from build123d import *

# Parameters (mm, degrees)
F0_R     = 5
F1_DEPTH = 10


with BuildPart() as f1:
    # F0 (on Top) → F1 (new body, symmetric)
    with BuildSketch(Plane.XY):
        with BuildLine():
            Line((25, 25), (25, 10))
            Line((25, 10), (-25, 10))
            ThreePointArc((-25, 10), (-35, 0), (-25, -10))
            Line((-25, -10), (25, -10))
            Line((25, -10), (25, -25))
            ThreePointArc((25, -25), (35, -35), (45, -25))
            Line((45, -25), (45, 25))
            ThreePointArc((45, 25), (35, 35), (25, 25))
        make_face()
        with Locations((35, -25)):
            Circle(F0_R, mode=Mode.SUBTRACT)
        with Locations((-25, 0)):
            Circle(F0_R, mode=Mode.SUBTRACT)
        with Locations((25, 0)):
            Circle(F0_R, mode=Mode.SUBTRACT)
        with Locations((35, 25)):
            Circle(F0_R, mode=Mode.SUBTRACT)
    extrude(amount=F1_DEPTH, both=True)


solid = f1.part
CAD build for the part. Positions are in the model's coordinates, mm. A direction names the side the tool comes from. Give positions to 0.01 mm unless a question says otherwise; leave off trailing zeros. Loops run counter-clockwise (first coordinate to the right, second up) from the corner with the lowest first, then second, coordinate; pieces in that order, holes last. Notation, with made-up numbers: M -29,49.5 L -10,49.5 A36 cw -10,86.5 Z; hole C -15,2.25 d3. An arc over 180 degrees is marked long. One line per question, with ' | ' between items. Start each with the question number.
1. Saw through at B-B on y = -21. Give the cut face in (x, z), plus the area to 3 significant figures.
2. Saw through at C-C on x = 21.5. Give the cut face in (y, z), plus the area to 3 significant figures.
3. Probe L1, parallel to Y at x = -25, z = 3.25; L2, parallel to X at y = -1, z = 2.75; L3, parallel to Y at x = 29.5, z = 7.25. List the from-to ranges inside material, lowest first. Write a range as from..to.
4. Flat gauge pins, fed straight in: pin 1 (4.5 mm diameter, centred on y = -19, z = -0.5, fed in from -X); pin 2 (8 mm diameter, centred on x = 1, z = -7.5, fed in from +Y); pin 3 (10 mm diameter, centred on x = 1.5, z = 0.5, fed in from -Y). Where does each tip first touch, or does it go through?
5. Two-plate mould, pull along Y, no slides. Class faces 4 (the face through (-35, 0, 0)), 5 (the face through (31, 22, 0)), 6 (the face through (25, 18, 0)), 7 (the face through (31, -28, 0)): pulls with the +Y half, pulls with the -Y half, needs draft (parallel to the pull), parting line crosses it, or undercut.
6. Saw through at A-A on y = 0. Give the cut face in (x, z), plus the area to 3 significant figures.
7. 3-axis set-ups, long thin cutter, end or side, ignore diameter. For faces 1 (the face through (0, -10, 0)), 2 (the face through (45, 0, 0)), 3 (the face through (0, 10, 0)): which of +Z, -Z, +X, -X, +Y, -Y reach the whole face in a straight line?
8. Saw through at D-D on z = 6.75. Give the cut face in (x, y).
Result sheet:
1) outline: M 25,-10 L 32,-10 L 32,10 L 25,10 Z; M 38,-10 L 45,-10 L 45,10 L 38,10 Z | area: 280 mm^2
2) outline: M -10,-10 L -3.57,-10 L -3.57,10 L -10,10 Z; M 3.57,-10 L 10,-10 L 10,10 L 3.57,10 Z | area: 257 mm^2
3) L1: y = -10..-5, 5..10 | L2: x = -34.95..-29.9, -20.1..20.1, 29.9..45 | L3: y = -33.35..-2.18, 2.18..33.35
4) pin 1: stops at x = 25 | pin 2: stops at y = 10 | pin 3: stops at y = -10
5) face 4: parting line crosses it | face 5: undercut | face 6: needs draft | face 7: undercut
6) outline: M -35,-10 L -30,-10 L -30,10 L -35,10 Z; M -20,-10 L 20,-10 L 20,10 L -20,10 Z; M 30,-10 L 45,-10 L 45,10 L 30,10 Z | area: 1,200 mm^2
7) face 1: +Z, -Z, -X, -Y | face 2: +Z, -Z, +X, +Y, -Y | face 3: +Z, -Z, -X, +Y
8) outline: M -25,-10 L 25,-10 L 25,-25 A10 ccw 45,-25 L 45,25 A10 ccw 25,25 L 25,10 L -25,10 A10 ccw Z; hole C -25,0 d10; hole C 25,0 d10; hole C 35,-25 d10; hole C 35,25 d10
